Check sheet for the drawn part. Datum: minimum x, y, z corner. Units: mm. A direction names the side the tool comes from. Round coordinates to 2 decimals unless told otherwise and drop trailing zeros. Write each loop counter-clockwise with the first axis right and the second up, starting at its lowest first coordinate (ties: lowest second). Pieces come first, ordered by that corner, then holes. Notation, with made-up numbers: (14.5, -0.5) -> (31.5, -0.5) arc R11 cw to (31.5, 10.5) -> close; hole circle Ø2 at (65, 57.25). An arc over 180 degrees is marked (long way). One line per item, written item: value. Start each with the question number.
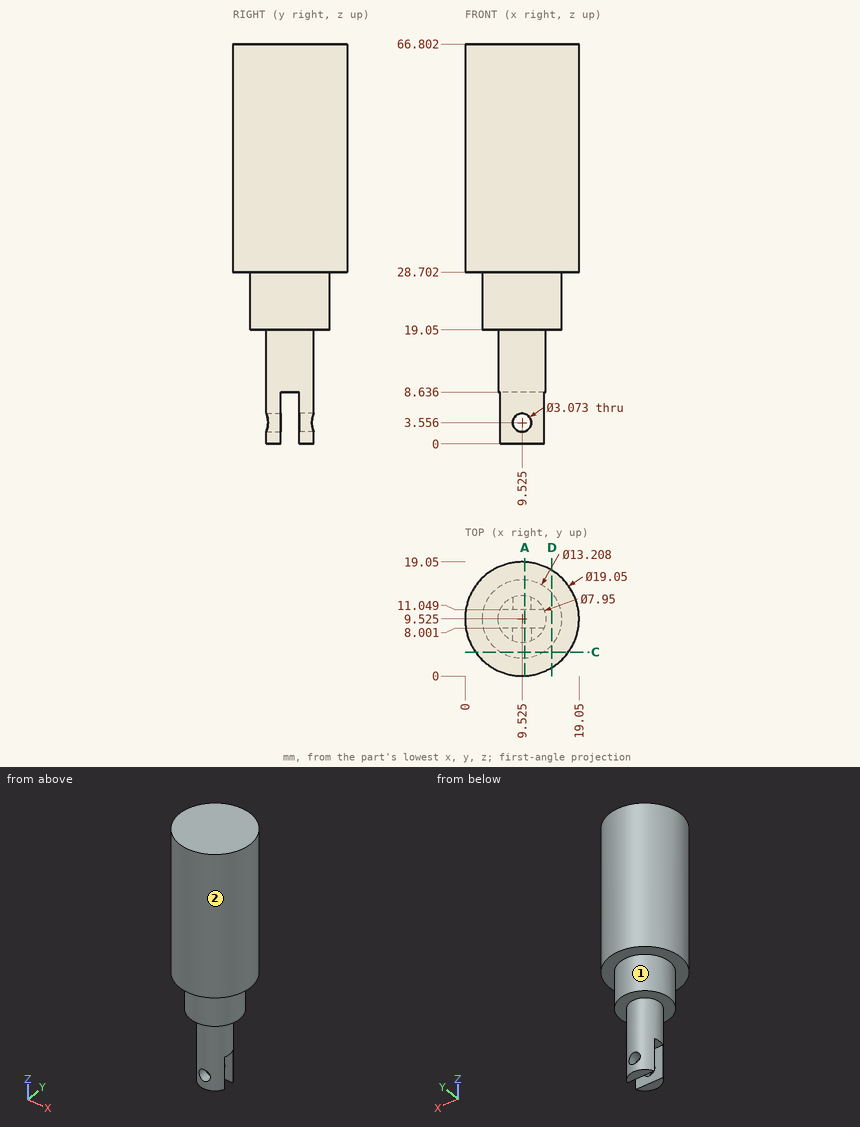
1. Material ranges on probe 1 along Z at (x, y) = (5.75, 15); probe 2 along Z at (x, y) = (11.5, 10.5); probe 3 along X at (y, z) = (9, 54) (1 decimal), recorded low to high.
2. Cross-section at A-A (x = 10). Give the number of separate pieces and of enclosed holes in the cut face, plus the area to 3 significant figures.
3. Depth check by flat-ended pin: pin 1 Ø5 at (x, z) = (9.525, 3.556) entering from +Y; pin 2 Ø1.5 at (x, z) = (5.5, 18.5) entering from -Y (1 decimal); pin 3 Ø3 at (x, z) = (2.5, 23) entering from -Y. Enter the tip coordinate at first touch or a pass-through.
4. Cross-section at D-D (x = 14.5). Record the cut outline in (y, z), plus the area to 3 significant figures.
5. Access from +Z, -Z, +X, -X, +Y, -Y to the whole of each face (thin tool, end or side, straight path). Record for the marked faces 1 and 2.
6. Cross-section at C-C (y = 4). Record the cut outline in (x, z), plus the area to 3 significant figures.
Working result:
1. probe 1: z = 28.7 to 66.8
1. probe 2: z = 8.64 to 66.8
1. probe 3: x = 0 to 19
2. separate pieces: 3
2. enclosed holes: 0
2. area: 962 mm^2
3. pin 1: stops at y = 13.5
3. pin 2: stops at y = 3.9
3. pin 3: stops at y = 5.91
4. outline: (1.4, 28.7) -> (5.18, 28.7) -> (5.18, 19.05) -> (13.87, 19.05) -> (13.87, 28.7) -> (17.65, 28.7) -> (17.65, 66.8) -> (1.4, 66.8) -> close
4. area: 703 mm^2
5. face 1: -Z
5. face 2: +Z, -Z
6. outline: (1.77, 28.7) -> (5.91, 28.7) -> (5.91, 19.05) -> (13.14, 19.05) -> (13.14, 28.7) -> (17.28, 28.7) -> (17.28, 66.8) -> (1.77, 66.8) -> close
6. area: 661 mm^2
